from build123d import *

# Parameters (mm, degrees)
CROQUIS1_R              = 40
DISCO_DEPTH             = 5
CORTAR_EXTRUIR1_DEPTH   = 10
SALIENTE_EXTRUIR5_START = -10
CROQUIS7_R              = 45
CROQUIS7_R_2            = 40
SALIENTE_EXTRUIR5_DEPTH = 10
CROQUIS8_R              = 41
CORTAR_EXTRUIR2_DEPTH   = 5


with BuildPart() as part:
    # Croquis1 → Disco (new body)
    with BuildSketch(Plane.XY):
        Circle(CROQUIS1_R)
    extrude(amount=DISCO_DEPTH)

    # Croquis6 → Cortar-Extruir1 (cut)
    with BuildSketch(Plane.XY.offset(5)):
        with BuildLine():
            Line((-5.25, 0), (-5.25, -30))
            ThreePointArc((-5.25, -30), (0, -35.25), (5.25, -30))
            Line((5.25, -30), (5.25, 0))
            ThreePointArc((5.25, 0), (0, 5.25), (-5.25, 0))
        make_face()
        with BuildLine():
            Line((2.625, 4.54663337), (-23.355762114, 19.54663337))
            ThreePointArc((-23.355762114, 19.54663337), (-30.527395483, 17.625), (-28.605762114, 10.45336663))
            Line((-28.605762114, 10.45336663), (-2.625, -4.54663337))
            ThreePointArc((-2.625, -4.54663337), (4.54663337, -2.625), (2.625, 4.54663337))
        make_face()
        with BuildLine():
            Line((2.625, -4.54663337), (28.605762114, 10.45336663))
            ThreePointArc((28.605762114, 10.45336663), (30.527395483, 17.625), (23.355762114, 19.54663337))
            Line((23.355762114, 19.54663337), (-2.625, 4.54663337))
            ThreePointArc((-2.625, 4.54663337), (-4.54663337, -2.625), (2.625, -4.54663337))
        make_face()
    extrude(amount=-CORTAR_EXTRUIR1_DEPTH, mode=Mode.SUBTRACT)

    # Croquis7 → Saliente-Extruir5 (add)
    with BuildSketch(Plane.XY.offset(5).offset(SALIENTE_EXTRUIR5_START)):
        Circle(CROQUIS7_R)
        Circle(CROQUIS7_R_2, mode=Mode.SUBTRACT)
    extrude(amount=SALIENTE_EXTRUIR5_DEPTH)

    # Croquis8 → Cortar-Extruir2 (cut)
    with BuildSketch(Plane(origin=(0, 0, -5), x_dir=(-1, 0, 0), z_dir=(0, 0, -1))):
        Circle(CROQUIS8_R)
    extrude(amount=-CORTAR_EXTRUIR2_DEPTH, mode=Mode.SUBTRACT)


solid = part.part
Work out the finished part from the listing and answer in its coordinate system (mm). A direction names the side the tool comes from. Coordinates: 2 decimals unless noted, no trailing zeros. Loops run counter-clockwise (first coordinate to the right, second up) from the corner with the lowest first, then second, coordinate; pieces in that order, holes last. Notation, with made-up numbers: (89, 39) -> (132, 39) arc R9 cw to (132, 54) -> close; hole circle Ø2 at (43.5, 6.5). An arc over 180 degrees is marked (long way). Answer as CSV lines item,"result".
1) For a pull along X with two mould halves and no side action, classify faces 1 (the face through (16.764, 3.617, 2.535)), 2 (the face through (20.765, -39.923, -0.07)), 3 (the face through (-1, 11, 5)) as released by +X, released by -X, zero draft, split by the parting line, or undercut.
A:
face 1,"undercut"
face 2,"split by the parting line"
face 3,"zero draft"
2) For faces 4 (the face through (-5.25, -16, 3)), 5 (the face through (-10, -40, -5)), 6 (the face through (9, -40, -3)), determine the directions among +Z, -Z, +X, -X, +Y, -Y from which every point of the face is accessible in a straight line to the end or side of a thin tool.
A:
face 4,"+Z, -Z"
face 5,"-Z, +X, -X, +Y, -Y"
face 6,"-Z"
3) The part is cut by section B-B (x = 7.5). Give the vertices of the cut face in (y, z), and give its area (3 significant figures).
A:
outline,"(-44.37, -5) -> (-40.31, -5) -> (-40.31, 0) -> (-1.73, 0) -> (-1.73, 5) -> (-44.37, 5) -> close; (10.39, 0) -> (40.31, 0) -> (40.31, -5) -> (44.37, -5) -> (44.37, 5) -> (10.39, 5) -> close"
area,"424 mm²"
4) The part is cut by section C-C (y = 15). Give the vertices of the cut face in (x, z).
A:
outline,"(-42.43, -5) -> (-38.16, -5) -> (-38.16, 0) -> (-31.23, 0) -> (-31.23, 5) -> (-42.43, 5) -> close; (-15.48, 0) -> (15.48, 0) -> (15.48, 5) -> (-15.48, 5) -> close; (31.23, 0) -> (38.16, 0) -> (38.16, -5) -> (42.43, -5) -> (42.43, 5) -> (31.23, 5) -> close"
5) Flat-ended cylindrical pins translate along their axes: pin 1 (1.5 mm diameter, centred on x = 33, z = -1, fed in from +Y); pin 2 (12 mm diameter, centred on x = 1, y = -11, fed in from -Z); pin 3 (4 mm diameter, centred on y = -18, z = 2, fed in from -X). Find the tip coordinate at first contact, or state that the pin passes through.
A:
pin 1,"stops at y = 31.38"
pin 2,"stops at z = 0"
pin 3,"stops at x = -42.06"
6) The part is cut by section A-A (y = 0). Give the vertices of the cut face in (x, z), and give its area (3 significant figures).
A:
outline,"(-45, -5) -> (-41, -5) -> (-41, 0) -> (-10.5, 0) -> (-10.5, 5) -> (-45, 5) -> close; (10.5, 0) -> (41, 0) -> (41, -5) -> (45, -5) -> (45, 5) -> (10.5, 5) -> close"
area,"385 mm²"
7) Straight lines are drawn through the part: probe 1 along Y at (x, z) = (0, -1.25); probe 2 along Z at (x, y) = (-0.5, 16.5); probe 3 along Y at (x, z) = (-36.5, -1.25). For each, find the intervals that lie inside material, in ascending order.
A:
probe 1,"y = -45 to -41, 41 to 45"
probe 2,"z = 0 to 5"
probe 3,"y = -26.32 to -18.67, 18.67 to 26.32"
